The model under review builds one solid part; all positions refer to its coordinate system, in mm. Face numbers are marked on the shaded views. A direction names the side the tool comes from. Round coordinates to 2 decimals unless told otherwise and drop trailing zeros. Write each loop counter-clockwise with the first axis right and the second up, starting at its lowest first coordinate (ties: lowest second). Pieces come first, ordered by that corner, then holes.
Item 1: Add section B-B (z = -1). Give the boundary of the cut face in (x, y), plus the area to 3 significant figures.
Item 2: Add section A-A (x = -5.05). Give the boundary of the cut face in (y, z), plus the area to 3 significant figures.
Item 3: Add section D-D (x = -7). Give the boundary of the cut face in (y, z).
Item 4: Add section C-C (y = -6.5). Give the boundary of the cut face in (x, z).
Item 5: Clearance check with flat-ended pins moving along their axes: pin 1 Ø1 at (x, y) = (-6, -7) entering from -Z; pin 2 Ø1.5 at (y, z) = (-6, -4) entering from +X. State where each tip first meets the part, or that it passes through.
Item 6: Draft analysis for pull direction Y (two halves, no side actions). For the marked faces 1, 2, 3 and 4, state which applies: +Y half, -Y half, draft (parallel to the pull), parting line (faces both ways), or undercut.
Item 7: Machinability: for the marked faces 5 and 6, which of the approach directions +Z, -Z, +X, -X, +Y, -Y give a long, thin tool a straight path to every point of the face, cutting with its end or side? Answer none if there is none.
Item 8: To check wall thickness, follow L1, parallel to Z at x = -6.6, y = -4.25 (3 decimals); L2, parallel to X at y = -8, z = -3. State the ranges of each line that lie inside material, in increasing order.
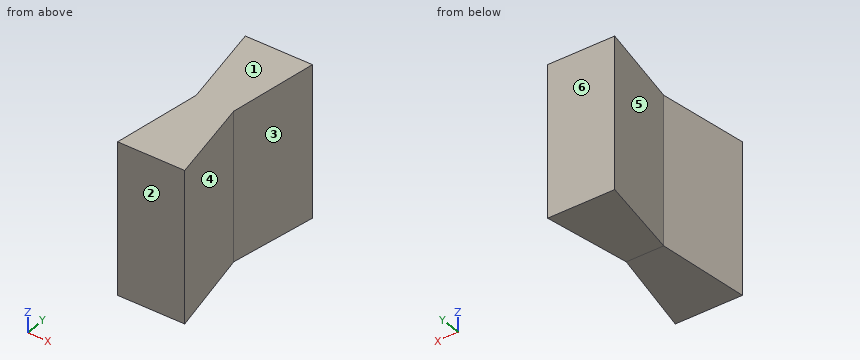
Autodesk Inventor part; units mm, degrees
ref_plane "Work Plane1" through (-10, -8, -5.5) normal (0, 0, -1) x (0, 1, 0)
ref_plane "YZ Plane" through (0, 0, 0) normal (1, 0, 0) x (0, 1, 0)
ref_plane "XZ Plane" through (0, 0, 0) normal (0, 1, 0) x (-1, 0, 0)
sketch "Sketch1" plane through (0, 0, 0) normal (0, 0, 1) x (1, 0, 0)
  line L0 (10, -8) -> (-10, -8)
  line L1 (-7, -8) -> (-7.6667, -12)
  line L2 (-7.6667, -12) -> (-4.3333, -12)
  line L3 (-4.3333, -12) -> (-5, -8)
  line L4 (-6, -8) -> (-6.0726, -4.2007)
  line L5 (-6, -8) -> (-6.8, -8)
  line L6 (-6, -8) -> (-5.2, -8)
  line L7 (-6.8, -8) -> (-7.4332, -4.2007)
  line L8 (-7.4332, -4.2007) -> (-6.0726, -4.2007)
  line L9 (-5.2, -8) -> (-4.5668, -4.2007)
  line L10 (-4.5668, -4.2007) -> (-6.0726, -4.2007)
  line L11 (-6, -8) -> (-6.0726, -11.7993)
  line L12 (-6.8, -8) -> (-7.4332, -11.7993)
  line L13 (-7.4332, -11.7993) -> (-6.0726, -11.7993)
  line L14 (-5.2, -8) -> (-4.5668, -11.7993)
  line L15 (-4.5668, -11.7993) -> (-6.0726, -11.7993)
  line L16 (-7, -8) -> (-7.6667, -4)
  line L17 (-7.6667, -4) -> (-4.3333, -4)
  line L18 (-4.3333, -4) -> (-5, -8)
  point P0 (0, 0)
  point P1 (-8, -8)
  point P2 (-5.2, -8)
  dimension "d2" = 3.8
  dimension "d3" = 0.8
  dimension "d4" = 0.8
ref_plane "Work Plane1" through (-10, -8, -5.5) normal (0, 0, -1) x (0, 1, 0)
extrude "Extrusion1" add sketch "Sketch1" against normal blind 7 contours L14 L15 L11 L0 | L0 L4 L10 L9 | L11 L13 L12 L0 | L0 L7 L8 L4
ref_plane "Work Plane2" through (-10, -8, 0) normal (-1, 0, 0) x (0, 1, 0)
sketch "Sketch2" plane through (-10, -8, 0) normal (-1, 0, 0) x (0, 1, 0)
  line L0 (3.7993, 0) -> (3.7993, 7)
  line L1 (0, 0) -> (0, 7)
  line L2 (-3.7993, 0) -> (-3.7993, 7)
  line L3 (15, 7) -> (0, 6.5)
  line L4 (0, 7) -> (3.7993, 7)
  line L5 (3.7993, 7) -> (0, 7)
  line L6 (-3.7993, 0) -> (-3.7993, 7)
  line L7 (-15, 7) -> (0, 6.5)
  line L8 (0, 7) -> (-3.7993, 7)
  point P0 (8, 0)
  point P1 (-3.7993, 6.6266)
  point P2 (3.7993, 6.6266)
extrude "Extrusion2" cut sketch "Sketch2" against normal through all
properties part number "key_3DPrint"
Numbers:
1. outline: (-7.43, -11.8) - (-4.57, -11.8) - (-5.2, -8) - (-4.57, -4.2) - (-7.43, -4.2) - (-6.8, -8) - close
1. area: 17.0 mm2
2. outline: (-11.8, -6.63) - (-8.9, -6.53) - (-8.9, 0) - (-11.8, 0) - close; (-7.1, -6.53) - (-4.2, -6.63) - (-4.2, 0) - (-7.1, 0) - close
2. area: 38.1 mm2
3. outline: (-11.8, -6.63) - (-9.2, -6.54) - (-9.2, 0) - (-11.8, 0) - close; (-6.8, -6.54) - (-4.2, -6.63) - (-4.2, 0) - (-6.8, 0) - close
4. outline: (-7.05, -6.55) - (-4.95, -6.55) - (-4.95, 0) - (-7.05, 0) - close
5. pin 1: stops at z = -6.55
5. pin 2: stops at x = -4.74
6. face 1: draft
6. face 2: -Y half
6. face 3: undercut
6. face 4: undercut
7. face 5: +Z, -Z, -X
7. face 6: +Z, -Z, +X, -X, +Y
8. L1: z = -6.625 to 0
8. L2: x = -6.8 to -5.2
